Drawing for the job (mm, zero at the part's lowest x, y, z). Coordinates: 2 decimals unless noted, no trailing zeros. Order: outer loops, then holes, each group sorted by start corner. A loop starts at its lowest first (then second) coordinate and runs counter-clockwise, first axis right, second up.
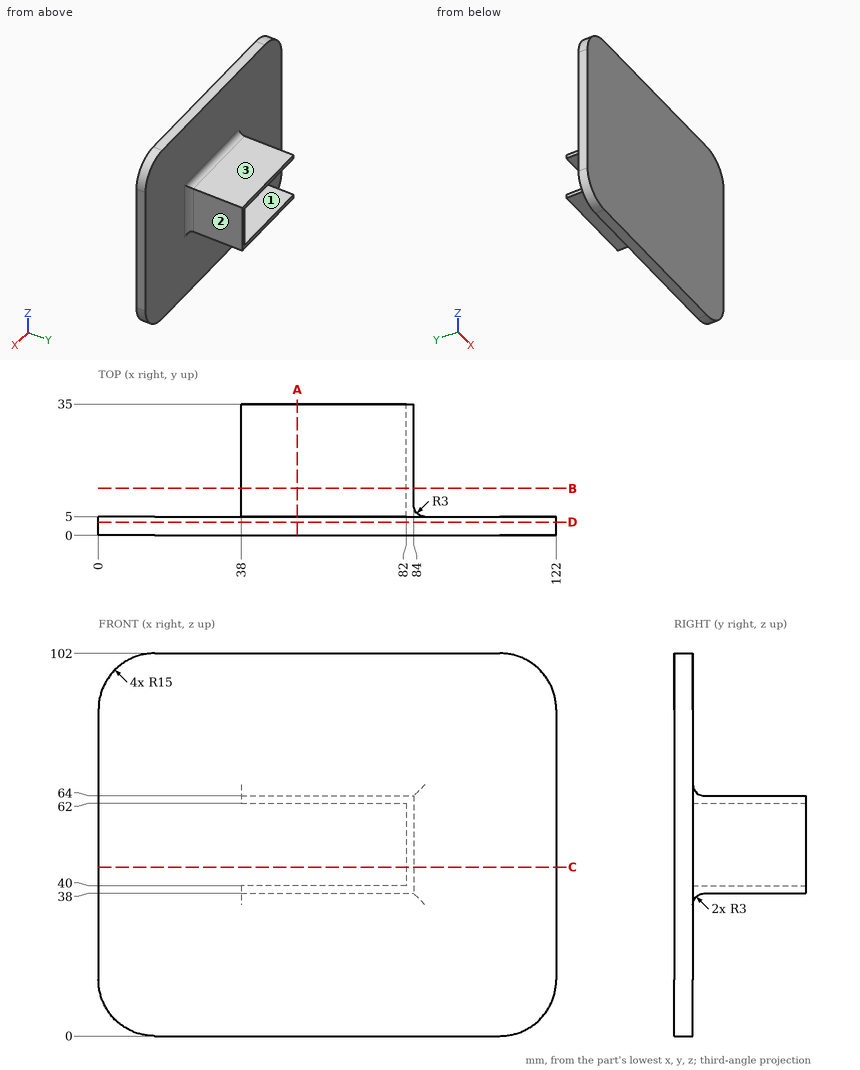
(1) Slice it at D-D, the plane y = 3.5. Give the cut face in (x, z).
(2) Slice it at C-C, the plane z = 45. Give the cut face in (x, y), then the cut area to 3 significant figures.
(3) Pull direction Z, two halves, no side cores. Call the marked faces 1, 2 and 3: +Z half, -Z half, draft (parallel to the pull), parting line (faces both ways), or undercut.
(4) Slice it at A-A, the plane x = 53. Give the cut face in (y, z), then the cut area to 3 significant figures.
(5) Probe line 1 (Z direction, x = 52, y = 13); line 2 (Y direction, x = 99, z = 30); line 3 (X direction, y = 18, z = 55). List the from-to ranges inside material, lowest first.
(6) Drop flat-ended pins along their axis: pin 1 (10 mm diameter, centred on x = 98, z = 46.5, fed in from +Y); pin 2 (5.5 mm diameter, centred on y = 24.5, z = 37, fed in from -X); pin 3 (2 mm diameter, centred on x = 105, z = 69.5, fed in from -Y). Give the stop position or say it passes through.
(7) Slice it at B-B, the plane y = 12.5. Give the cut face in (x, z), then the cut area to 3 significant figures.
Here are the results:
1. outline: (0, 15) arc R15 ccw to (15, 0) - (107, 0) arc R15 ccw to (122, 15) - (122, 87) arc R15 ccw to (107, 102) - (15, 102) arc R15 ccw to (0, 87) - close
2. outline: (0, 0) - (122, 0) - (122, 5) - (87, 5) arc R3 cw to (84, 8) - (84, 35) - (82, 35) - (82, 5) - (0, 5) - close
2. area: 672 mm2
3. face 1: undercut
3. face 2: draft
3. face 3: +Z half
4. outline: (0, 0) - (5, 0) - (5, 35) arc R3 cw to (8, 38) - (35, 38) - (35, 40) - (5, 40) - (5, 62) - (35, 62) - (35, 64) - (8, 64) arc R3 cw to (5, 67) - (5, 102) - (0, 102) - close
4. area: 634 mm2
5. line 1: z = 38 to 40, 62 to 64
5. line 2: y = 0 to 5
5. line 3: x = 82 to 84
6. pin 1: stops at y = 5
6. pin 2: stops at x = 38
6. pin 3: stops at y = 0
7. outline: (38, 38) - (84, 38) - (84, 64) - (38, 64) - (38, 62) - (82, 62) - (82, 40) - (38, 40) - close
7. area: 228 mm2
